Source: CAD feature listing. Evaluate the final solid. Frame: model axes, mm. Coordinates: 2 decimals unless noted, no trailing zeros. Order: outer loops, then holes, each group sorted by start corner. A loop starts at its lowest first (then second) coordinate and runs counter-clockwise, first axis right, second up.
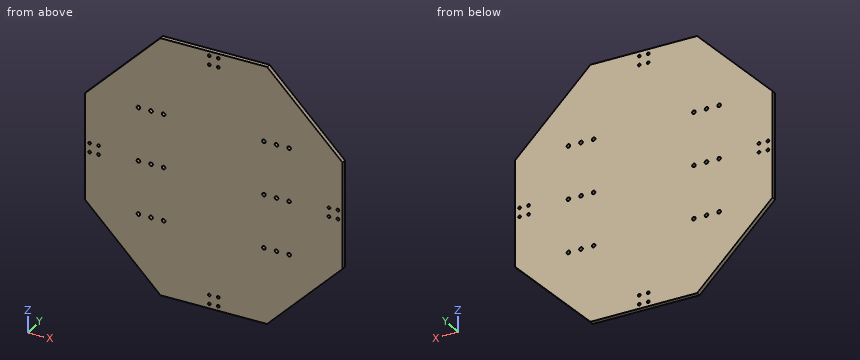
```python
from build123d import *

# Parameters (mm, degrees)
SKETCH_1_R          = 1.5
EXTRUDE_1_DEPTH     = 5
SKETCH_2_R          = 2
CUT_EXTRUDE_1_DEPTH = 10


with BuildPart() as part:
    # 스케치1 → 보스-돌출1 (new body)
    with BuildSketch(Plane(origin=(0, 0, 0), x_dir=(1, 0, 0), z_dir=(0, 1, 0))):
        Polygon((59.481067557, -143.6), (143.6, -59.481067557), (143.6, 59.481067557), (59.481067557, 143.6), (-59.481067557, 143.6), (-143.6, 59.481067557), (-143.6, -59.481067557), (-59.481067557, -143.6), align=None)
        with Locations((-5, 138.54)):
            Circle(SKETCH_1_R, mode=Mode.SUBTRACT)
        with Locations((-5, 128.54)):
            Circle(SKETCH_1_R, mode=Mode.SUBTRACT)
        with Locations((5, 128.54)):
            Circle(SKETCH_1_R, mode=Mode.SUBTRACT)
        with Locations((5, 138.54)):
            Circle(SKETCH_1_R, mode=Mode.SUBTRACT)
        with Locations((138.54, 5)):
            Circle(SKETCH_1_R, mode=Mode.SUBTRACT)
        with Locations((128.54, 5)):
            Circle(SKETCH_1_R, mode=Mode.SUBTRACT)
        with Locations((128.54, -5)):
            Circle(SKETCH_1_R, mode=Mode.SUBTRACT)
        with Locations((138.54, -5)):
            Circle(SKETCH_1_R, mode=Mode.SUBTRACT)
        with Locations((5, -138.54)):
            Circle(SKETCH_1_R, mode=Mode.SUBTRACT)
        with Locations((5, -128.54)):
            Circle(SKETCH_1_R, mode=Mode.SUBTRACT)
        with Locations((-5, -128.54)):
            Circle(SKETCH_1_R, mode=Mode.SUBTRACT)
        with Locations((-5, -138.54)):
            Circle(SKETCH_1_R, mode=Mode.SUBTRACT)
        with Locations((-138.54, -5)):
            Circle(SKETCH_1_R, mode=Mode.SUBTRACT)
        with Locations((-128.54, -5)):
            Circle(SKETCH_1_R, mode=Mode.SUBTRACT)
        with Locations((-128.54, 5)):
            Circle(SKETCH_1_R, mode=Mode.SUBTRACT)
        with Locations((-138.54, 5)):
            Circle(SKETCH_1_R, mode=Mode.SUBTRACT)
    extrude(amount=EXTRUDE_1_DEPTH)

    # 스케치2 → 컷-돌출1 (cut)
    with BuildSketch(Plane(origin=(0, 5, 0), x_dir=(1, 0, 0), z_dir=(0, 1, 0))):
        with Locations((-56, 0)):
            Circle(SKETCH_2_R)
        with Locations((-56, 59.482135114)):
            Circle(SKETCH_2_R)
        with Locations((-56, -59.482135114)):
            Circle(SKETCH_2_R)
        with Locations((70, 0)):
            Circle(SKETCH_2_R)
        with Locations((70, 59.482135114)):
            Circle(SKETCH_2_R)
        with Locations((70, -59.482135114)):
            Circle(SKETCH_2_R)
        with Locations((-70, -59.482135114)):
            Circle(SKETCH_2_R)
        with Locations((-70, 59.482135114)):
            Circle(SKETCH_2_R)
        with Locations((-70, 0)):
            Circle(SKETCH_2_R)
        with Locations((56, -59.482135114)):
            Circle(SKETCH_2_R)
        with Locations((56, 59.482135114)):
            Circle(SKETCH_2_R)
        with Locations((56, 0)):
            Circle(SKETCH_2_R)
        with Locations((-84, 0)):
            Circle(SKETCH_2_R)
        with Locations((-84, 59.482135114)):
            Circle(SKETCH_2_R)
        with Locations((-84, -59.482135114)):
            Circle(SKETCH_2_R)
        with Locations((84, -59.482135114)):
            Circle(SKETCH_2_R)
        with Locations((84, 59.482135114)):
            Circle(SKETCH_2_R)
        with Locations((84, 0)):
            Circle(SKETCH_2_R)
    extrude(amount=-CUT_EXTRUDE_1_DEPTH, mode=Mode.SUBTRACT)


solid = part.part
```
Q1. Section query C-C on y = 2.65. Give the number of separate pieces and of enclosed holes in the cut face, plus the area to 3 significant figures.
Solutions:
separate pieces: 1
enclosed holes: 34
area: 68,000 mm2
Q2. Pin query (flat end, axial travel): P1, Ø2, axis at y = 2.5, z = 101.5, coming from the -X side; P2, Ø3, axis at y = 1, z = -101, coming from the -X side; P3, Ø2, axis at y = 2.5, z = 108, coming from the -X side. Return the tip coordinate at first contact, or that it passes through.
Solutions:
P1: stops at x = -102.58
P2: stops at x = -103.58
P3: stops at x = -96.08
Q3. Section query A-A on x = 112.5. Output: boundary loops of the cut face in (y, z).
Solutions:
outline: (0, -90.58) - (5, -90.58) - (5, 90.58) - (0, 90.58) - close
Q4. Section query B-B on z = -115. Output: boundary loops of the cut face in (x, y), plus the area to 3 significant figures.
Solutions:
outline: (-88.08, 0) - (88.08, 0) - (88.08, 5) - (-88.08, 5) - close
area: 881 mm2
Q5. Material intervals for line 1 along Z through (x, y) = (56, 3.65); line 2 along X through (y, z) = (1.95, -5), sorted ascending.
Solutions:
line 1: z = -143.6 to -61.48, -57.48 to -2, 2 to 57.48, 61.48 to 143.6
line 2: x = -143.6 to -140.04, -137.04 to -130.04, -127.04 to 127.04, 130.04 to 137.04, 140.04 to 143.6
